The model under review builds one solid part; all positions refer to its coordinate system, in mm. A direction names the side the tool comes from. Coordinates: 2 decimals unless noted, no trailing zeros. Write each loop counter-clockwise with the first axis right and the second up, starting at its lowest first coordinate (ties: lowest second). Pieces come first, ordered by that corner, then holes. Notation, with made-up numbers: (-0.75, 13) - (30.25, 13) arc R26 ccw to (30.25, 47) - close; hole circle Ø11 at (45.25, 73.5). An arc over 180 degrees is marked (long way). Put each result on its own line as item: value. Start each with the question number.
Item 1: Consider section A-A on x = 4.05. Give the boundary of the cut face in (y, z), then the cut area to 3 significant figures.
Item 2: Consider section C-C on z = 12.25. Give the boundary of the cut face in (x, y), then the cut area to 3 significant figures.
Item 3: Consider section D-D on x = 2.4. Give the boundary of the cut face in (y, z), then the cut area to 3 significant figures.
Item 4: Consider section B-B on y = 1.05. Give the boundary of the cut face in (x, z).
Item 5: Mouldability with a two-part tool opening along X and no side actions: class faces 1 (the face through (2.972, 1, 8)), 2 (the face through (5.055, 1, 8)), 3 (the face through (2.5, 1.6, 15.24)) as pulls with the +X half, pulls with the -X half, needs draft (parallel to the pull), parting line crosses it, or undercut.
Item 6: Machinability: for faces 4 (the face through (1.4, 2.388, 2.5)), 5 (the face through (3.6, 2.083, 7.8)), 6 (the face through (2.5, 2.515, 7.5)), which of the approach directions +Z, -Z, +X, -X, +Y, -Y give a long, thin tool a straight path to every point of the face, cutting with its end or side? Answer none if there is none.
Item 7: To check wall thickness, follow L1, parallel to X at y = 1.2, z = 13; L2, parallel to Z at x = 3.9, y = 2.2; L3, parallel to Y at x = 1.4, z = 8.5. State the ranges of each line that lie inside material, in increasing order. Write a range as [from, to].
```python
from build123d import *

# Parameters (mm, degrees)
SKETCH1_W           = 5.0546
SKETCH1_H           = 2.5146
BOSS_EXTRUDE1_DEPTH = 15.24
SKETCH2_W           = 1.143
SKETCH2_H           = 1.143
CUT_EXTRUDE1_DEPTH  = 16.24
CHAMFER1_SIZE       = 0.254
SKETCH3_W           = 0.762
SKETCH3_H           = 0.762
SKETCH3_H_2         = 1.524
CUT_EXTRUDE2_DEPTH  = 1.27
SKETCH4_W           = 1.651
SKETCH4_H           = 1.651
CUT_EXTRUDE3_DEPTH  = 15.732
SKETCH6_W           = 1.143
SKETCH6_H           = 0.762
CUT_EXTRUDE5_DEPTH  = 0.4318
SKETCH7_W           = 0.508
SKETCH7_H           = 7.62
CUT_EXTRUDE6_DEPTH  = 0.762
SKETCH8_W           = 0.8128
SKETCH8_H           = 0.0762
CUT_EXTRUDE7_DEPTH  = 0.127


with BuildPart() as part:
    # Sketch1 → Boss-Extrude1 (new body)
    with BuildSketch(Plane.XY):
        with Locations((2.5273, 1.2573)):
            Rectangle(SKETCH1_W, SKETCH1_H)
    extrude(amount=BOSS_EXTRUDE1_DEPTH)

    # Sketch2 → Cut-Extrude1 (cut, through all)
    with BuildSketch(Plane(origin=(0, 0, 0), x_dir=(-1, 0, 0), z_dir=(0, 0, -1))):
        with Locations((-3.7973, 1.2573)):
            Rectangle(SKETCH2_W, SKETCH2_H)
        with Locations((-1.2573, 1.2573)):
            Rectangle(SKETCH2_W, SKETCH2_H)
    extrude(amount=-CUT_EXTRUDE1_DEPTH, mode=Mode.SUBTRACT)

    # Chamfer1
    chamfer1_edges = [part.edges().sort_by_distance(p)[0] for p in [
        (4.3688, 1.2573, 0),
        (3.7973, 0.6858, 0),
        (3.2258, 1.2573, 0),
        (3.7973, 1.8288, 0),
        (1.8288, 1.2573, 0),
        (1.2573, 0.6858, 0),
        (0.6858, 1.2573, 0),
        (1.2573, 1.8288, 0),
    ]]
    chamfer(chamfer1_edges, length=CHAMFER1_SIZE)

    # Sketch3 → Cut-Extrude2 (cut)
    with BuildSketch(Plane(origin=(0, 2.5146, 0), x_dir=(1, 0, 0), z_dir=(0, 1, 0))):
        with Locations((4.1656, -14.097)):
            Rectangle(SKETCH3_W, SKETCH3_H)
        with Locations((1.6256, -14.097)):
            Rectangle(SKETCH3_W, SKETCH3_H)
        with Locations((4.1656, -7.62)):
            Rectangle(SKETCH3_W, SKETCH3_H_2)
        with Locations((1.6256, -7.62)):
            Rectangle(SKETCH3_W, SKETCH3_H_2)
    extrude(amount=-CUT_EXTRUDE2_DEPTH, mode=Mode.SUBTRACT)

    # Sketch4 → Cut-Extrude3 (cut, through all)
    with BuildSketch(Plane.XY.offset(0.508)):
        with Locations((1.2573, 1.2573)):
            Rectangle(SKETCH4_W, SKETCH4_H)
        with Locations((3.7973, 1.2573)):
            Rectangle(SKETCH4_W, SKETCH4_H)
    extrude(amount=CUT_EXTRUDE3_DEPTH, mode=Mode.SUBTRACT)

    # Sketch6 → Cut-Extrude5 (cut)
    with BuildSketch(Plane.XZ):
        with Locations((1.5113, 14.859)):
            Rectangle(SKETCH6_W, SKETCH6_H)
        with Locations((4.0513, 14.859)):
            Rectangle(SKETCH6_W, SKETCH6_H)
    extrude(amount=-CUT_EXTRUDE5_DEPTH, mode=Mode.SUBTRACT)

    # Sketch7 → Cut-Extrude6 (cut)
    with BuildSketch(Plane.XZ):
        with Locations((2.4638, 3.81)):
            Rectangle(SKETCH7_W, SKETCH7_H)
    extrude(amount=-CUT_EXTRUDE6_DEPTH, mode=Mode.SUBTRACT)

    # Sketch8 → Cut-Extrude7 (cut)
    with BuildSketch(Plane(origin=(0, 2.5146, 0), x_dir=(1, 0, 0), z_dir=(0, 1, 0))):
        Polygon((1.397, -1.143), (0.889, -3.3274), (1.905, -3.3274), align=None)
        with Locations((1.397, -3.8481)):
            Rectangle(SKETCH8_W, SKETCH8_H)
    extrude(amount=-CUT_EXTRUDE7_DEPTH, mode=Mode.SUBTRACT)


solid = part.part
```
Report:
1. outline: (0, 0) - (0.43, 0) - (0.69, 0.25) - (0.69, 0.51) - (0.43, 0.51) - (0.43, 14.48) - (0, 14.48) - close; (1.83, 0.25) - (2.08, 0) - (2.51, 0) - (2.51, 6.86) - (2.08, 6.86) - (2.08, 0.51) - (1.83, 0.51) - close; (2.08, 8.38) - (2.51, 8.38) - (2.51, 13.72) - (2.08, 13.72) - close; (2.08, 14.48) - (2.51, 14.48) - (2.51, 15.24) - (2.08, 15.24) - close
1. area: 12.0 mm²
2. outline: (0, 0) - (5.05, 0) - (5.05, 2.51) - (0, 2.51) - close; hole (0.43, 0.43) - (2.08, 0.43) - (2.08, 2.08) - (0.43, 2.08) - close; hole (2.97, 0.43) - (4.62, 0.43) - (4.62, 2.08) - (2.97, 2.08) - close
2. area: 7.26 mm²
3. outline: (0, 7.62) - (0.76, 7.62) - (0.76, 0) - (2.51, 0) - (2.51, 15.24) - (0, 15.24) - close
3. area: 32.5 mm²
4. outline: (0, 0) - (0.43, 0) - (0.69, 0.25) - (0.69, 0.51) - (0.43, 0.51) - (0.43, 15.24) - (0, 15.24) - close; (1.83, 0.25) - (2.08, 0) - (2.97, 0) - (3.23, 0.25) - (3.23, 0.51) - (2.97, 0.51) - (2.97, 15.24) - (2.08, 15.24) - (2.08, 0.51) - (1.83, 0.51) - close; (4.37, 0.25) - (4.62, 0) - (5.05, 0) - (5.05, 15.24) - (4.62, 15.24) - (4.62, 0.51) - (4.37, 0.51) - close
5. face 1: undercut
5. face 2: pulls with the +X half
5. face 3: needs draft
6. face 4: +Y
6. face 5: +Z
6. face 6: +Z, -Z, +X, -X, +Y
7. L1: [0, 0.43], [2.08, 2.97], [4.62, 5.05]
7. L2: [0, 6.86], [8.38, 13.72], [14.48, 15.24]
7. L3: [0, 0.43], [2.08, 2.51]
